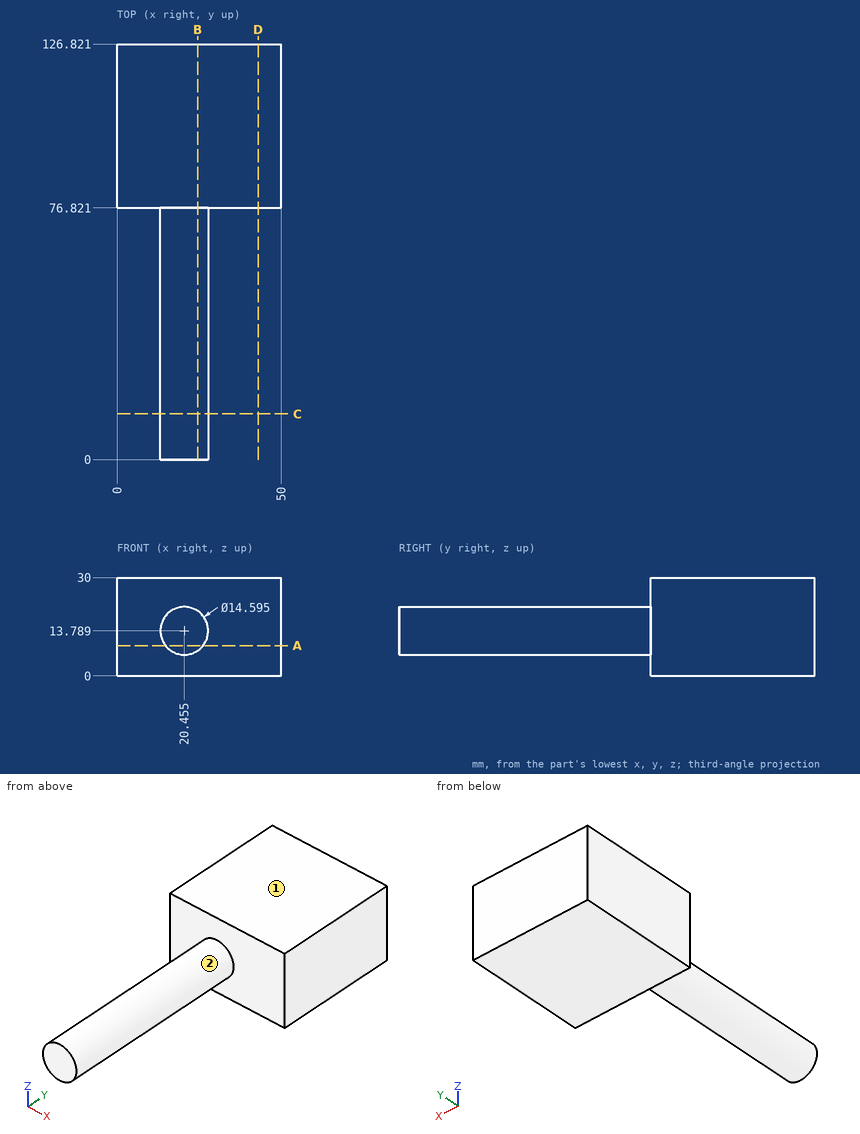
Drawing for the job (mm, zero at the part's lowest x, y, z). A direction names the side the tool comes from. Give positions to 0.01 mm unless a question says otherwise; leave off trailing zeros. Loops run counter-clockwise (first coordinate to the right, second up) from the corner with the lowest first, then second, coordinate; pieces in that order, holes last. Notation, with made-up numbers: (-17, -5) - (28, -5) arc R3 ccw to (28, -1) - close; hole circle Ø10 at (38.5, 14). An arc over 180 degrees is marked (long way). Write item = value, one per line. Start each with the question number.
1) Band-saw the part on C-C on y = 14. Give the cut face in (x, z) (1 decimal), plus the area to 3 significant figures.
2) Tool access for the marked faces 1 and 2: list every direction of +Z, -Z, +X, -X, +Y, -Y with a clear straight run to the whole face (end or side of a thin tool).
3) Band-saw the part on B-B on x = 24.5. Give the cut face in (y, z) (1 decimal).
4) Band-saw the part on D-D on x = 43. Give the cut face in (y, z).
5) Band-saw the part on A-A on z = 9.25. Give the cut face in (x, y), plus the area to 3 significant figures.
6) Drop flat-ended pins along their axis: pin 1 Ø1.5 at (x, y) = (17.5, 14.5) entering from +Z (1 decimal); pin 2 Ø12 at (y, z) = (41, 6.5) entering from +X; pin 3 Ø8 at (y, z) = (66, 23.5) entering from +X. Give the stop position or say it passes through.
7) Probe probe 1 along Y at (x, z) = (38.5, 1.5); probe 2 along X at (y, z) = (22, 16.25) (1 decimal); probe 3 along Z at (x, y) = (18, 28.5). List the from-to ranges inside material, lowest first. Write a range as from..to.
Final values:
q1.outline = circle Ø14.6 at (20.5, 13.8)
q1.area = 167 mm²
q2.face_1 = +Z, +X, -X, +Y, -Y
q2.face_2 = -Y
q3.outline = (0, 7.7) - (76.8, 7.7) - (76.8, 0) - (126.8, 0) - (126.8, 30) - (76.8, 30) - (76.8, 19.9) - (0, 19.9) - close
q4.outline = (76.82, 0) - (126.82, 0) - (126.82, 30) - (76.82, 30) - close
q5.outline = (0, 76.82) - (14.74, 76.82) - (14.74, 0) - (26.17, 0) - (26.17, 76.82) - (50, 76.82) - (50, 126.82) - (0, 126.82) - close
q5.area = 3,380 mm²
q6.pin_1 = 20.7
q6.pin_2 = 27.64
q6.pin_3 = 25
q7.probe_1 = 76.82..126.82
q7.probe_2 = 13.6..27.3
q7.probe_3 = 6.92..20.66
